Design review of the part built by this model. Coordinates are the model's own, in mm. A direction names the side the tool comes from. Give positions to 0.01 mm unless a question says otherwise; leave off trailing zeros. Order: outer loops, then holes, each group sorted by start corner. A loop starts at its lowest first (then second) coordinate and runs counter-clockwise, first axis right, second up.
```python
from build123d import *

# Parameters (mm, degrees)
SKETCH2_R                                       = 1.6
CUT_EXTRUDE1_DEPTH                              = 19.350749304
CSK_FOR_M3_FLAT_HEAD_MACHINE_SCREW1_D           = 2.8
CSK_FOR_M3_FLAT_HEAD_MACHINE_SCREW1_CSINK_D     = 6.5
CSK_FOR_M3_FLAT_HEAD_MACHINE_SCREW1_CSINK_ANGLE = 90
FILLET1_R                                       = 0.5
FILLET2_R                                       = 0.25


with BuildPart() as part:
    # Sketch1 → Revolve1 (revolve)
    with BuildSketch(Plane.XY, mode=Mode.PRIVATE) as revolve1_sk:
        Polygon((0, 8.5), (10.025, 8.5), (10.025, 1.5), (11.5, 1.5), (11.5, 0), (0, 0), align=None)
    revolve(revolve1_sk.sketch.rotate(Axis((0, 0, 0), (0, 1, 0)), 90), axis=Axis((0, 0, 0), (0, 1, 0)))

    # Sketch2 → Cut-Extrude1 (cut, through all)
    with BuildSketch(Plane.XZ):
        with Locations(Location((0, 7, 0), (0, 0, 270))):
            Circle(SKETCH2_R)
        with Locations(Location((7, 0, 0), (0, 0, 270))):
            Circle(SKETCH2_R)
        with Locations(Location((0, -7, 0), (0, 0, 270))):
            Circle(SKETCH2_R)
        with Locations(Location((-7, 0, 0), (0, 0, 270))):
            Circle(SKETCH2_R)
    extrude(amount=-CUT_EXTRUDE1_DEPTH, mode=Mode.SUBTRACT)

    # CSK for M3 Flat Head Machine Screw1 (through all)
    with Locations(Plane(origin=(0, 0, 7), x_dir=(0, 0, -1), z_dir=(0, -1, 0))):
        with Locations((0, 0), (7, 7), (14, 0), (7, -7)):
            CounterSinkHole(CSK_FOR_M3_FLAT_HEAD_MACHINE_SCREW1_D / 2, CSK_FOR_M3_FLAT_HEAD_MACHINE_SCREW1_CSINK_D / 2, counter_sink_angle=CSK_FOR_M3_FLAT_HEAD_MACHINE_SCREW1_CSINK_ANGLE)

    # Fillet1
    fillet1_edges = [part.edges().sort_by_distance(p)[0] for p in [
        (0, 8.5, 10.025),
    ]]
    fillet(fillet1_edges, radius=FILLET1_R)

    # Fillet2
    fillet2_edges = [part.edges().sort_by_distance(p)[0] for p in [
        (0, 0, 11.5),
        (0, 1.5, 11.5),
    ]]
    fillet(fillet2_edges, radius=FILLET2_R)


solid = part.part
```
1. Draft analysis for pull direction Z (two halves, no side actions). For faces 3 (the face through (-8.56, 5.03, 0.35)), 4 (the face through (-11.4, 0.7, 1.5)), 5 (the face through (7, 1.5, -8)), state which applies: pulls with the +Z half, pulls with the -Z half, needs draft (parallel to the pull), parting line crosses it, or undercut.
Recorded:
face 3: undercut
face 4: parting line crosses it
face 5: needs draft
2. For pin 1 (5 mm diameter, centred on y = 6.5, z = 8.5, fed in from -X); pin 2 (1.5 mm diameter, centred on y = 6.5, z = -5.5, fed in from -X); pin 3 (5 mm diameter, centred on y = 7, z = -6.5, fed in from -X), all flat-tipped, find the tip position at first contact; note any pin that passes through.
Recorded:
pin 1: stops at x = -8.03
pin 2: stops at x = -8.83
pin 3: stops at x = -9.19
3. Take a section at A-A (x = 0). State the section outline as (y, z) points (3 decimals).
Recorded:
outline: (0, -11.25) arc R0.25 ccw to (0.25, -11.5) - (1.25, -11.5) arc R0.25 ccw to (1.5, -11.25) - (1.5, -10.025) - (8, -10.025) arc R0.5 ccw to (8.5, -9.525) - (8.5, -8.6) - (1.65, -8.6) - (0, -10.25) - close; (0, -3.75) - (1.65, -5.4) - (8.5, -5.4) - (8.5, 5.4) - (1.65, 5.4) - (0, 3.75) - close; (0, 10.25) - (1.65, 8.6) - (8.5, 8.6) - (8.5, 9.525) arc R0.5 ccw to (8, 10.025) - (1.5, 10.025) - (1.5, 11.25) arc R0.25 ccw to (1.25, 11.5) - (0.25, 11.5) arc R0.25 ccw to (0, 11.25) - close
4. Machinability: for faces 1 (the face through (0.07, 5.03, 8.6)), 2 (the face through (6.1, 4.704, 7.955)), which of the approach directions +Z, -Z, +X, -X, +Y, -Y give a long, thin tool a straight path to every point of the face, cutting with its end or side? Answer none if there is none.
Recorded:
face 1: +Y, -Y
face 2: +Y
5. For line 1 along X through (y, z) = (4, 0) (3 decimals); line 2 along Y through (x, z) = (5, -10); line 3 along X through (y, z) = (5.25, -7), list the stretches that pass through material, from the lowest coordinate up.
Recorded:
line 1: x = -10.025 to -8.6, -5.4 to 5.4, 8.6 to 10.025
line 2: y = 0 to 1.5
line 3: x = -7.18 to -1.6, 1.6 to 7.18
6. Take a section at B-B (y = 3). State the section outline as (x, z) points (3 decimals).
Recorded:
outline: circle Ø20.05 at (0, 0); hole circle Ø3.2 at (-7, 0); hole circle Ø3.2 at (0, -7); hole circle Ø3.2 at (0, 7); hole circle Ø3.2 at (7, 0)
